from build123d import *

# Parameters (mm, degrees)
ESQUISSE1_W             = 13
ESQUISSE1_H             = 9.5
BOSS_EXTRU_1_DEPTH      = 50
ESQUISSE2_R             = 1.75
ENL_V_MAT_EXTRU_1_DEPTH = 500
ESQUISSE3_W             = 50
ESQUISSE3_H             = 61.5
BOSS_EXTRU_2_DEPTH      = 4
ESQUISSE4_R             = 1.75
ENL_V_MAT_EXTRU_2_DEPTH = 33.5
CONG_2_R                = 3
ENL_V_START             = -5
ESQUISSE5_R             = 1.75
ENL_V_MAT_EXTRU_3_DEPTH = 5


with BuildPart() as part:
    # Esquisse1 → Boss.-Extru.1 (new body)
    with BuildSketch(Plane.XY):
        with Locations((6.5, 4.75)):
            Rectangle(ESQUISSE1_W, ESQUISSE1_H)
    extrude(amount=BOSS_EXTRU_1_DEPTH)

    # Esquisse2 → Enlèv. mat.-Extru.1 (cut)
    with BuildSketch(Plane(origin=(0, 9.5, 0), x_dir=(1, 0, 0), z_dir=(0, 1, 0))):
        with Locations(Location((8.7, -40, 0), (0, 0, 270))):
            Circle(ESQUISSE2_R)
        with BuildLine():
            Line((6.95, -10), (6.95, -9))
            ThreePointArc((6.95, -9), (8.7, -7.25), (10.45, -9))
            Line((10.45, -9), (10.45, -10))
            ThreePointArc((10.45, -10), (8.7, -11.75), (6.95, -10))
        make_face()
    extrude(amount=-ENL_V_MAT_EXTRU_1_DEPTH, mode=Mode.SUBTRACT)

    # Esquisse3 → Boss.-Extru.2 (add)
    with BuildSketch(Plane.ZY):
        with Locations((25, -21.25)):
            Rectangle(ESQUISSE3_W, ESQUISSE3_H)
    extrude(amount=BOSS_EXTRU_2_DEPTH)

    # Esquisse4 → Enlèv. mat.-Extru.2 (cut)
    with BuildSketch(Plane(origin=(0, 0, 0), x_dir=(0, 0, -1), z_dir=(1, 0, 0))):
        with BuildLine():
            Line((-44.209372712, -10), (-50, -10))
            Line((-50, -10), (-50, -52))
            Line((-50, -52), (0, -52))
            Line((0, -52), (0, -10))
            Line((0, -10), (-5.790627288, -10))
            ThreePointArc((-5.790627288, -10), (-25, -1), (-44.209372712, -10))
        make_face()
        with Locations((-45, -6)):
            Circle(ESQUISSE4_R)
        with Locations((-5, -6)):
            Circle(ESQUISSE4_R)
    extrude(amount=-ENL_V_MAT_EXTRU_2_DEPTH, mode=Mode.SUBTRACT)

    # Congé2
    # the kernel refuses this fillet: 3 mm, written as the material it takes off along each edge
    with BuildSketch(Plane(origin=(13, 9.5, -7.5), x_dir=(0, -1, 0), z_dir=(0, 0, 1))) as cong_2_piece_1:
        with BuildLine():
            CenterArc((CONG_2_R, -CONG_2_R), CONG_2_R, 90, 90)
            Line((0, -CONG_2_R), (0, 0))
            Line((0, 0), (CONG_2_R, 0))
        make_face()
    extrude(amount=65, mode=Mode.SUBTRACT)

    # Esquisse5 → Enlèv. mat.-Extru.3 (cut)
    # profile 1 of 4: a face of its own
    with BuildSketch(Plane(origin=(0, 0, 0), x_dir=(-1, 0, 0), z_dir=(0, -1, 0)).offset(ENL_V_START)):
        Polygon((-5.8, -38.325684219), (-8.7, -36.651368439), (-11.6, -38.325684219), (-11.6, -41.674315781), (-8.7, -43.348631561), (-5.8, -41.674315781), align=None)
        with Locations(Location((-8.7, -40, 0), (0, 0, 222.024627579))):
            Circle(ESQUISSE5_R, mode=Mode.SUBTRACT)
    # profile 2 of 4: a face of its own
    with BuildSketch(Plane(origin=(0, 0, 0), x_dir=(-1, 0, 0), z_dir=(0, -1, 0)).offset(ENL_V_START)):
        Polygon((-11.6, -7.325684219), (-11.6, -8.325684219), (-8.7, -6.651368439), (-5.8, -8.325684219), (-5.8, -7.325684219), (-8.7, -5.651368439), align=None)
    # profile 3 of 4: a face of its own
    with BuildSketch(Plane(origin=(0, 0, 0), x_dir=(-1, 0, 0), z_dir=(0, -1, 0)).offset(ENL_V_START)):
        Polygon((-11.6, -10.674315781), (-11.6, -11.674315781), (-8.7, -13.348631561), (-5.8, -11.674315781), (-5.8, -10.674315781), (-8.7, -12.348631561), align=None)
    # profile 4 of 4: a face of its own
    with BuildSketch(Plane(origin=(0, 0, 0), x_dir=(-1, 0, 0), z_dir=(0, -1, 0)).offset(ENL_V_START)):
        Polygon((-11.6, -8.325684219), (-11.6, -10.674315781), (-8.7, -12.348631561), (-5.8, -10.674315781), (-5.8, -8.325684219), (-8.7, -6.651368439), align=None)
        with BuildLine():
            ThreePointArc((-10.45, -9), (-8.7, -7.25), (-6.95, -9))
            Line((-6.95, -9), (-6.95, -10))
            ThreePointArc((-6.95, -10), (-8.7, -11.75), (-10.45, -10))
            Line((-10.45, -10), (-10.45, -9))
        make_face(mode=Mode.SUBTRACT)
    extrude(amount=ENL_V_MAT_EXTRU_3_DEPTH, mode=Mode.SUBTRACT)


solid = part.part
Could you check a few things on this model? Use its own coordinates, in mm. A direction names the side the tool comes from. Coordinates: 2 decimals unless noted, no trailing zeros. Order: outer loops, then holes, each group sorted by start corner. A loop starts at its lowest first (then second) coordinate and runs counter-clockwise, first axis right, second up.
Q1. Will these pins go through, and if not, where does the flat tip stop? pin 1 (5.5 mm diameter, centred on y = -6, z = 45, fed in from +X); pin 2 (4 mm diameter, centred on x = 8.7, z = 40, fed in from -Y); pin 3 (3 mm diameter, centred on y = -6, z = 5, fed in from -X); pin 4 (1.1 mm diameter, centred on y = 8.5, z = 9.5, fed in from +X).
Q2. Please list where these lines run through material, in increasing order: L1, parallel to Z at x = 8.7, y = 7.45; L2, parallel to Y at x = -2.05, z = 45; L3, parallel to Z at x = 11, y = 3.
Q3. Suppose I cut it at D-D on x = 8. Please give me the cut outline in (y, z).
Q4. Which directions (+Z, -Z, +X, -X, +Y, -Y) give clear straight access to the entire face, cutting with the end or side of a thin tool? Please do faces 1 (the flat face through (6.95, 7.3, 9.5)), 2 (the flat face through (13, 3, 25)), 3 (the flat face through (5.8, 3, 40)).
Q5. Suppose I cut it at C-C on y = -6. Please give me the cut outline in (x, z), and give its area (3 significant figures).
Q6. Suppose I cut it at A-A on y = 1.5. Please give me the cut outline in (x, z), and give its area (3 significant figures).
Q7. Thinking about a two-plate mould opening in X: for faces 4 (the flat face through (6, 0, 25)), 5 (the flat face through (-4, 2, 25)), 6 (the flat face through (10.17, 2.54, 12.5)), which applies, released by +X, released by -X, zero draft, split by the parting line, or undercut?
Q8. Suppose I cut it at B-B on z = 45. Please give me the cut outline in (x, y).
Answer:
1. pin 1: stops at x = 0
1. pin 2: stops at y = 5
1. pin 3: passes through
1. pin 4: stops at x = 12.63
2. L1: z = 0 to 7.25, 11.75 to 38.25, 41.75 to 50
2. L2: y = -10 to -7.75, -4.25 to 9.5
2. L3: z = 0 to 6.98, 12.02 to 37.98, 42.02 to 50
3. outline: (0, 0) - (9.5, 0) - (9.5, 7.4) - (5, 7.4) - (5, 6.06) - (0, 6.06) - close; (0, 12.94) - (5, 12.94) - (5, 11.6) - (9.5, 11.6) - (9.5, 38.4) - (5, 38.4) - (5, 37.06) - (0, 37.06) - close; (0, 42.94) - (5, 42.94) - (5, 41.6) - (9.5, 41.6) - (9.5, 50) - (0, 50) - close
4. face 1: +Y, -Y
4. face 2: +Z, -Z, +X, +Y, -Y
4. face 3: -Y
5. outline: (-4, 0) - (0, 0) - (0, 3.25) - (-4, 3.25) - close; (-4, 6.75) - (0, 6.75) - (0, 10) - (-4, 10) - close; (-4, 40) - (0, 40) - (0, 43.25) - (-4, 43.25) - close; (-4, 46.75) - (0, 46.75) - (0, 50) - (-4, 50) - close
5. area: 52.0 mm2
6. outline: (-4, 0) - (13, 0) - (13, 50) - (-4, 50) - close; hole (5.8, 7.33) - (8.7, 5.65) - (11.6, 7.33) - (11.6, 11.67) - (8.7, 13.35) - (5.8, 11.67) - close; hole (5.8, 38.33) - (8.7, 36.65) - (11.6, 38.33) - (11.6, 41.67) - (8.7, 43.35) - (5.8, 41.67) - close
6. area: 786 mm2
7. face 4: zero draft
7. face 5: released by -X
7. face 6: undercut
8. outline: (-4, -10) - (0, -10) - (0, -7.75) - (-4, -7.75) - close; (-4, -4.25) - (0, -4.25) - (0, 0) - (13, 0) - (13, 6.5) arc R3 ccw to (10, 9.5) - (-4, 9.5) - close
